Study the drawing (mm; zero at the part's minimum x, y, z) and answer. Coordinates: 2 decimals unless noted, no trailing zeros. Order: outer loops, then holes, each group sorted by start corner. A loop starts at its lowest first (then second) coordinate and runs counter-clockwise, first axis right, second up.
1. Find the intervals of material crossed by probe 1 along Y at (x, z) = (6.35, 0.9); probe 2 along Y at (x, z) = (9, 0.3); probe 3 along X at (y, z) = (3, 0.7), in increasing order.
2. Flat-ended cylindrical pins translate along their axes: pin 1 Ø1 at (x, z) = (18, 1.5) entering from -Y (1 decimal); pin 2 Ø1.7 at (x, z) = (8, 1.5) entering from -Y; pin 3 Ø1 at (y, z) = (1.5, 1.5) entering from -X. Find the tip coordinate at first contact, or state that the pin passes through.
3. The part is cut by section A-A, the plane x = 6.35. Give the vertices of the cut face in (y, z).
4. The part is cut by section B-B, the plane y = 50.8. Give the vertices of the cut face in (x, z) (1 decimal).
5. The part is cut by section C-C, the plane z = 0.95. Count the separate pieces of the cut face and the enclosed holes in it, then the cut area to 3 significant figures.
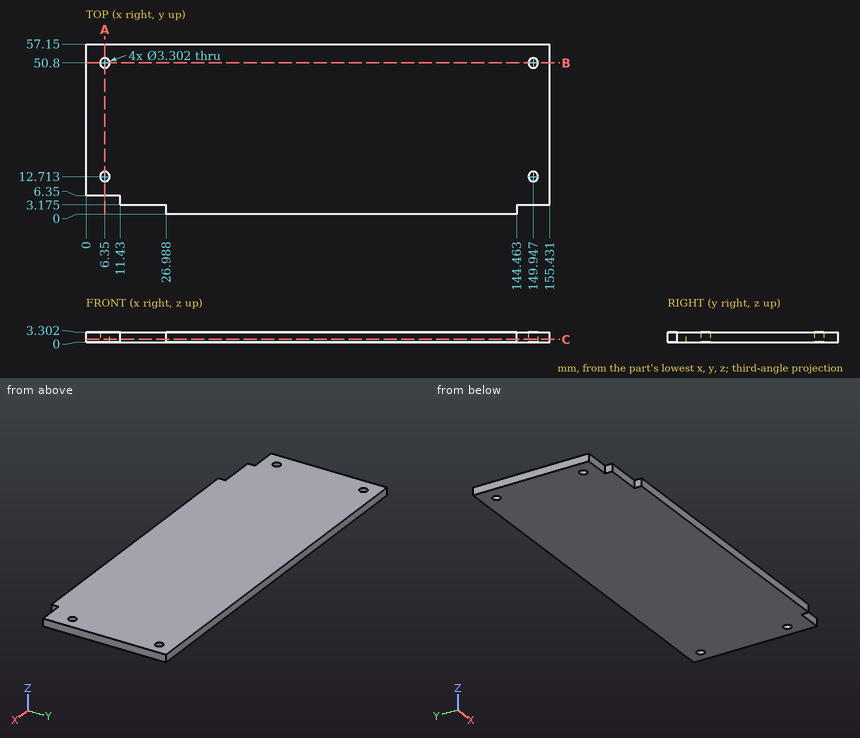
Geometry says:
1. probe 1: y = 6.35 to 11.06, 14.36 to 49.15, 52.45 to 57.15
1. probe 2: y = 6.35 to 57.15
1. probe 3: x = 26.99 to 144.46
2. pin 1: stops at y = 3.2
2. pin 2: stops at y = 6.35
2. pin 3: stops at x = 26.99
3. outline: (6.35, 0) - (11.06, 0) - (11.06, 3.3) - (6.35, 3.3) - close; (14.36, 0) - (49.15, 0) - (49.15, 3.3) - (14.36, 3.3) - close; (52.45, 0) - (57.15, 0) - (57.15, 3.3) - (52.45, 3.3) - close
4. outline: (0, 0) - (4.7, 0) - (4.7, 3.3) - (0, 3.3) - close; (8, 0) - (148.3, 0) - (148.3, 3.3) - (8, 3.3) - close; (151.6, 0) - (155.4, 0) - (155.4, 3.3) - (151.6, 3.3) - close
5. separate pieces: 1
5. enclosed holes: 4
5. area: 8,690 mm2
